CAD build for the part. Positions are in the model's coordinates, mm. A direction names the side the tool comes from. Give positions to 0.01 mm unless a question says otherwise; leave off trailing zeros. Order: outer loops, then holes, each group sorted by start corner. A loop starts at its lowest first (then second) coordinate and runs counter-clockwise, first axis right, second up.
from build123d import *

# Parameters (mm, degrees)
SKETCH2_W           = 203.2
SKETCH2_H           = 152.4
BOSS_EXTRUDE1_DEPTH = 152.4
SKETCH4_W           = 50.8
SKETCH4_H           = 101.6
CUT_EXTRUDE1_DEPTH  = 76.2
SKETCH5_W           = 25.4
SKETCH5_H           = 50.8
CUT_EXTRUDE2_DEPTH  = 76.2
SKETCH6_W           = 50.8
SKETCH6_H           = 25.4
CUT_EXTRUDE3_DEPTH  = 152.4
CUT_EXTRUDE4_DEPTH  = 76.2


with BuildPart() as part:
    # Sketch2 → Boss-Extrude1 (new body)
    with BuildSketch(Plane.XY):
        with Locations((101.6, 76.2)):
            Rectangle(SKETCH2_W, SKETCH2_H)
    extrude(amount=-BOSS_EXTRUDE1_DEPTH)

    # Sketch4 → Cut-Extrude1 (cut)
    with BuildSketch(Plane.XY):
        with Locations((25.4, 50.8)):
            Rectangle(SKETCH4_W, SKETCH4_H)
    extrude(amount=-CUT_EXTRUDE1_DEPTH, mode=Mode.SUBTRACT)

    # Sketch5 → Cut-Extrude2 (cut)
    with BuildSketch(Plane(origin=(0, 152.4, 0), x_dir=(1, 0, 0), z_dir=(0, 1, 0))):
        with Locations((12.7, 50.8)):
            Rectangle(SKETCH5_W, SKETCH5_H)
    extrude(amount=-CUT_EXTRUDE2_DEPTH, mode=Mode.SUBTRACT)

    # Sketch6 → Cut-Extrude3 (cut)
    with BuildSketch(Plane(origin=(203.2, 0, 0), x_dir=(0, 0, -1), z_dir=(1, 0, 0))):
        with Locations((50.8, 12.7)):
            Rectangle(SKETCH6_W, SKETCH6_H)
    extrude(amount=-CUT_EXTRUDE3_DEPTH, mode=Mode.SUBTRACT)

    # Sketch7 → Cut-Extrude4 (cut)
    with BuildSketch(Plane(origin=(0, 152.4, 0), x_dir=(1, 0, 0), z_dir=(0, 1, 0))):
        Polygon((152.4, 152.4), (152.4, 50.8), (101.6, 50.8), (101.6, 0), (203.2, 0), (203.2, 152.4), align=None)
    extrude(amount=-CUT_EXTRUDE4_DEPTH, mode=Mode.SUBTRACT)


solid = part.part
1. 3-axis set-ups, long thin cutter, end or side, ignore diameter. For faces 5 (the flat face through (127, 115, -50.8)), 6 (the flat face through (152.4, 115, -102)), 7 (the flat face through (48, 48, -76.2)), 8 (the flat face through (50.8, 61, -38)), 9 (the flat face through (128, 13, -25.4)): which of +Z, -Z, +X, -X, +Y, -Y reach the whole face in a straight line?
2. Saw through at D-D on x = 127.5. Give the cut face in (y, z).
3. Pin check, flat tips, straight feed: P1, Ø5, axis at x = 163, y = 20.5, coming from the +Z side; P2, Ø15, axis at x = 112, z = -47, coming from the -Y side; P3, Ø1, axis at y = 29, z = -42, coming from the -X side; P4, Ø15, axis at y = 118.5, z = -46, coming from the -X side. Stop position of each tip, or through.
4. Saw through at B-B on y = 14. Give the cut face in (x, z), plus the area to 3 significant figures.
5. Wall check: line 1 (Z direction, x = 23.5, y = 117.5); line 2 (X direction, y = 49.5, z = -46.5); line 3 (Y direction, x = 163.5, z = -46.5). Give the ranges that are in metal, low to high.
6. Saw through at C-C on z = -36. Give the cut face in (x, y), plus the area to 3 significant figures.
7. Mould opens along Z. For faces 1 (the flat face through (13, 127, -25.4)), 2 (the flat face through (100, 77, -152.4)), 3 (the flat face through (0, 75, -114)), 4 (the flat face through (100, 77, 0)) say: released by +Z, released by -Z, zero draft, split by the parting line, or undercut.
8. Saw through at A-A on x = 16. Give the cut face in (y, z), plus the area to 3 significant figures.
Reported:
1. face 5: +Z, +X, +Y
1. face 6: +Z, -Z, +X, +Y
1. face 7: -X, -Y
1. face 8: +Z, -X, -Y
1. face 9: +X, -X, -Y
2. outline: (0, -152.4) - (152.4, -152.4) - (152.4, -50.8) - (76.2, -50.8) - (76.2, 0) - (0, 0) - (0, -25.4) - (25.4, -25.4) - (25.4, -76.2) - (0, -76.2) - close
3. P1: stops at z = 0
3. P2: stops at y = 25.4
3. P3: stops at x = 50.8
3. P4: stops at x = 25.4
4. outline: (0, -152.4) - (203.2, -152.4) - (203.2, -76.2) - (0, -76.2) - close; (50.8, -25.4) - (203.2, -25.4) - (203.2, 0) - (50.8, 0) - close
4. area: 19,400 mm2
5. line 1: z = -152.4 to -76.2, -25.4 to 0
5. line 2: x = 50.8 to 203.2
5. line 3: y = 25.4 to 76.2
6. outline: (25.4, 101.6) - (50.8, 101.6) - (50.8, 25.4) - (203.2, 25.4) - (203.2, 76.2) - (101.6, 76.2) - (101.6, 152.4) - (25.4, 152.4) - close
6. area: 12,900 mm2
7. face 1: undercut
7. face 2: released by -Z
7. face 3: zero draft
7. face 4: released by +Z
8. outline: (0, -152.4) - (152.4, -152.4) - (152.4, -76.2) - (0, -76.2) - close; (101.6, -25.4) - (152.4, -25.4) - (152.4, 0) - (101.6, 0) - close
8. area: 12,900 mm2
